Here's how the part is built. I have some questions about the finished solid (model axes, mm). Face numbers are marked on the shaded views. Give positions to 0.01 mm unless a question says otherwise; leave off trailing zeros. Loops run counter-clockwise (first coordinate to the right, second up) from the corner with the lowest first, then second, coordinate; pieces in that order, holes last. Notation, with made-up numbers: (54, -5.5) -> (102, -5.5) arc R15 cw to (102, 14.5) -> close; hole circle Ø3 at (61, -33). An arc over 180 degrees is marked (long way). Answer in a Markdown table with one row per item. Add a question column.
Item 1: We'd pull the mould along X, two halves only. Please class the marked faces 1 and 2: released by +X, released by -X, zero draft, split by the parting line, or undercut.
Item 2: For P1, Ø10, axis at x = -13, y = -2, coming from the +Z side; P2, Ø1, axis at x = -4, y = -10, coming from the -Z side; P3, Ø4, axis at x = 10.5, y = 1, coming from the -Z side; P4, Ø1.5, axis at x = 14, y = 14, coming from the -Z side, each with a flat end and sliding along its axis, tell me the tip position at first contact or that it passes through.
Item 3: If we section it at A-A (z = 24.5): Write out the boundary of the cut face in (x, y).
Item 4: If I drill on line 1 (Z direction, x = 0, y = -0.75); line 2 (Z direction, x = 0, y = 5); line 3 (Z direction, x = 0, y = 6.5), over which ranges is the centre line in solid material (lowest first)?
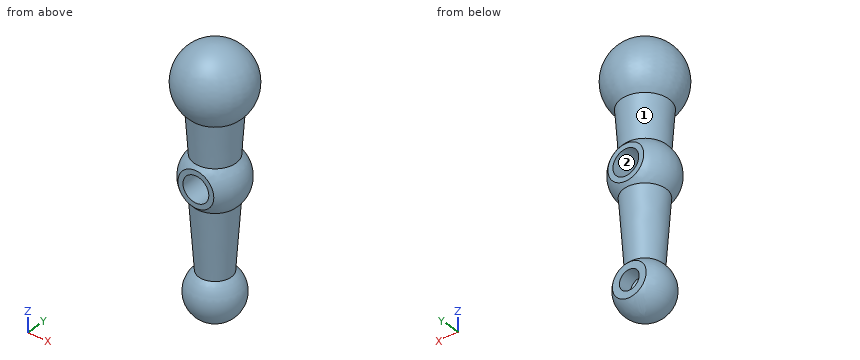
```python
from build123d import *

# Parameters (mm, degrees)
CUT_EXTRUDE1_DEPTH         = 73.608539
CUT_EXTRUDE1_DEPTH_BACK    = 73.608539
SKETCH2_R                  = 6.5
CUT_EXTRUDE7_DEPTH         = 73.608539
CUT_EXTRUDE7_DEPTH_BACK    = 12
F_10_0MM_DOWEL_HOLE1_D     = 10
F_10_0MM_DOWEL_HOLE1_DEPTH = 6.995697
F_10_0MM_DOWEL_HOLE1_TIP   = 3.004303


with BuildPart() as part:
    # Sketch1 → Revolve1 (revolve)
    with BuildSketch(Plane(origin=(0, 0, 0), x_dir=(0, 0, -1), z_dir=(1, 0, 0))):
        with BuildLine():
            Line((-63, 0), (68, 0))
            ThreePointArc((68, 0), (59.318672, 12.261691), (44.869373, 8.146803))
            Line((44.869373, 8.146803), (10.674844, 10.537918))
            ThreePointArc((10.674844, 10.537918), (0, 15), (-10.674844, 10.537918))
            Line((-10.674844, 10.537918), (-31.583592, 12))
            ThreePointArc((-31.583592, 12), (-51.422798, 16.815102), (-63, 0))
        make_face()
    revolve(axis=Axis((0, 0, 63), (0, 0, -1)))

    # Sketch2 → Cut-Extrude1 (cut, two sides: drawn at the far end of the back side and taken through both)
    with BuildSketch(Plane(origin=(0, 0, 0), x_dir=(1, 0, 0), z_dir=(0, 1, 0)).offset(-CUT_EXTRUDE1_DEPTH_BACK)):
        with Locations(Location((0, 0, 0), (0, 0, 270))):
            Circle(SKETCH2_R)
    extrude(amount=CUT_EXTRUDE1_DEPTH + CUT_EXTRUDE1_DEPTH_BACK, mode=Mode.SUBTRACT)

    # Sketch6 → Cut-Extrude7 (cut, two sides: drawn at the far end of the back side and taken through both)
    with BuildSketch(Plane(origin=(0, 0, 0), x_dir=(0, 0, -1), z_dir=(1, 0, 0)).offset(-CUT_EXTRUDE7_DEPTH_BACK)):
        with BuildLine():
            Line((6.5, 13.518506), (-6.5, 13.518506))
            ThreePointArc((-6.5, 13.518506), (-7.787102, 12.820337), (-9, 12))
            Line((-9, 12), (9, 12))
            ThreePointArc((9, 12), (7.787102, 12.820337), (6.5, 13.518506))
        make_face()
        with BuildLine():
            Line((9, -12), (-9, -12))
            ThreePointArc((-9, -12), (-7.787102, -12.820337), (-6.5, -13.518506))
            Line((-6.5, -13.518506), (6.5, -13.518506))
            ThreePointArc((6.5, -13.518506), (7.787102, -12.820337), (9, -12))
        make_face()
        with BuildLine():
            Line((46.5, 9.836158), (63.5, 9.836158))
            ThreePointArc((63.5, 9.836158), (55, 13), (46.5, 9.836158))
        make_face()
    extrude(amount=CUT_EXTRUDE7_DEPTH + CUT_EXTRUDE7_DEPTH_BACK, mode=Mode.SUBTRACT)

    # Ø10.0mm Dowel Hole1
    with Locations(Plane(origin=(0, 9.836158, -55), x_dir=(0, 0, 1), z_dir=(0, 1, 0))):
        with Locations((0, 0)):
            Hole(F_10_0MM_DOWEL_HOLE1_D / 2, depth=F_10_0MM_DOWEL_HOLE1_DEPTH)
            with Locations((0, 0, -(F_10_0MM_DOWEL_HOLE1_DEPTH + F_10_0MM_DOWEL_HOLE1_TIP / 2))):  # 118° drill point
                Cone(0, F_10_0MM_DOWEL_HOLE1_D / 2, F_10_0MM_DOWEL_HOLE1_TIP, mode=Mode.SUBTRACT)


solid = part.part
```
Recorded:
| question | item | result |
|---|---|---|
| 1 | face 1 | split by the parting line |
| 1 | face 2 | undercut |
| 2 | P1 | stops at z = 61.05 |
| 2 | P2 | stops at z = -62.97 |
| 2 | P3 | stops at z = -64.79 |
| 2 | P4 | passes through |
| 3 | outline | circle Ø23.01 at (0, 0) |
| 4 | line 1 | z = -67.98 to -6.5, 6.5 to 62.98 |
| 4 | line 2 | z = -67 to -60, -50 to -6.5, 6.5 to 62.29 |
| 4 | line 3 | z = -66.26 to -60, -50 to -6.5, 6.5 to 61.79 |
